from build123d import *

# Parameters (mm, degrees)
SKETCH2_R           = 3.175
BOSS_EXTRUDE1_DEPTH = 56.32
SKETCH3_R           = 2.794
BOSS_EXTRUDE2_DEPTH = 0.7366
SKETCH4_R           = 3.175
BOSS_EXTRUDE3_DEPTH = 2


with BuildPart() as part:
    # Sketch2 → Boss-Extrude1 (new body)
    with BuildSketch(Plane.XY):
        Circle(SKETCH2_R)
    boss_extrude1 = extrude(amount=BOSS_EXTRUDE1_DEPTH)

    # Sketch3 → Boss-Extrude2 (add)
    with BuildSketch(Plane.XY.offset(56.32)):
        Circle(SKETCH3_R)
    boss_extrude2 = extrude(amount=BOSS_EXTRUDE2_DEPTH)

    # Sketch4 → Boss-Extrude3 (add)
    with BuildSketch(Plane.XY.offset(57.0566)):
        Circle(SKETCH4_R)
    boss_extrude3 = extrude(amount=BOSS_EXTRUDE3_DEPTH)

    # Mirror1: Boss-Extrude1, Boss-Extrude2, Boss-Extrude3 across plane
    add(boss_extrude1.mirror(Plane.XY))
    add(boss_extrude2.mirror(Plane.XY))
    add(boss_extrude3.mirror(Plane.XY))


solid = part.part
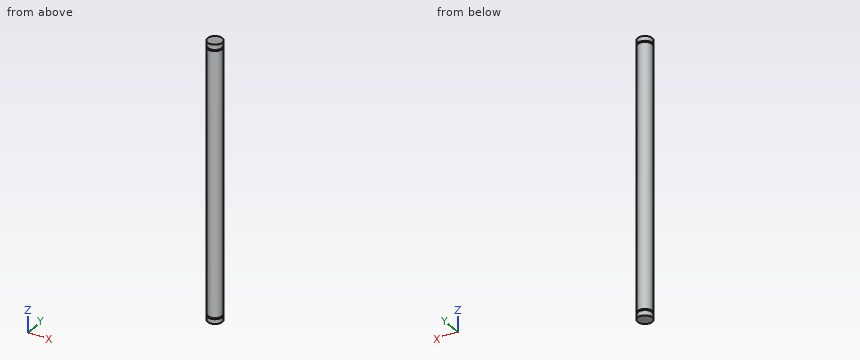
CAD build for the part. Positions are in the model's coordinates, mm. Give positions to 0.01 mm unless a question says otherwise; leave off trailing zeros. Order: outer loops, then holes, each group sorted by start corner. A loop starts at its lowest first (then second) coordinate and runs counter-clockwise, first axis right, second up. Notation, with made-up numbers: (7, 82.5) - (47, 82.5) arc R26 cw to (47, 119.5) - close; hole circle Ø1 at (39.5, -13.75). An arc over 180 degrees is marked (long way). Write each question's results on one line, items separated by ' | '.
1. Probe L1, parallel to Z at x = 2.75, y = -0.75; L2, parallel to Y at x = 1.5, z = 36.5; L3, parallel to X at y = -0.25, z = -1. List the from-to ranges inside material, lowest first. Write a range as from..to.
Calculated:
L1: z = -59.06..-57.06, -56.32..56.32, 57.06..59.06 | L2: y = -2.8..2.8 | L3: x = -3.17..3.17
2. Saw through at A-A on x = 1.5. List the corners of the cut face in (y, z), and give its area (3 significant figures).
Calculated:
outline: (-2.8, -59.06) - (2.8, -59.06) - (2.8, -57.06) - (2.36, -57.06) - (2.36, -56.32) - (2.8, -56.32) - (2.8, 56.32) - (2.36, 56.32) - (2.36, 57.06) - (2.8, 57.06) - (2.8, 59.06) - (-2.8, 59.06) - (-2.8, 57.06) - (-2.36, 57.06) - (-2.36, 56.32) - (-2.8, 56.32) - (-2.8, -56.32) - (-2.36, -56.32) - (-2.36, -57.06) - (-2.8, -57.06) - close | area: 660 mm2
3. Pin check, flat tips, straight feed: pin 1 (1 mm diameter, centred on x = -2, z = -46, fed in from +Y); pin 2 (1.5 mm diameter, centred on x = -1, z = -20, fed in from -Y). Stop position of each tip, or through.
Calculated:
pin 1: stops at y = 2.8 | pin 2: stops at y = -3.17
4. Saw through at B-B on z = 20. List the corners of the cut face in (x, y) (3 decimals), and give its area (3 significant figures).
Calculated:
outline: circle Ø6.35 at (0, 0) | area: 31.7 mm2
